Work out the finished part from the listing and answer in its coordinate system (mm). A direction names the side the tool comes from. Give positions to 0.01 mm unless a question says otherwise; leave off trailing zeros. Loops run counter-clockwise (first coordinate to the right, second up) from the corner with the lowest first, then second, coordinate; pieces in that order, holes last. Notation, with made-up numbers: M -24,-25 L 17,-25 A19 cw 17,-4 Z; hole C -21,82 d8. An arc over 180 degrees is marked long. Answer in a Markdown table with one row per item. Add a question column.
from build123d import *

# Parameters (mm, degrees)
BOSS_EXTRUDE1_DEPTH      = 28.5
SKETCH2_W                = 12
SKETCH2_H                = 11
SKETCH2_R                = 1.7
BOSS_EXTRUDE2_DEPTH      = 3
SKETCH3_W                = 19
SKETCH3_H                = 6
BOSS_EXTRUDE3_DEPTH      = 4
M3_CLEARANCE_HOLE1_D     = 3.2
M3_CLEARANCE_HOLE1_DEPTH = 4
FILLET1_R                = 3
M3_CLEARANCE_HOLE2_D     = 3.6
FILLET2_R                = 2


with BuildPart() as part:
    # Sketch1 → Boss-Extrude1 (new body)
    with BuildSketch(Plane.XY):
        with BuildLine():
            Line((-3.5, 44), (-3.5, 39.846580782))
            ThreePointArc((-3.5, 39.846580782), (0, 40), (3.5, 39.846580782))
            Line((3.5, 39.846580782), (3.5, 44))
            Line((3.5, 44), (-3.5, 44))
        make_face()
    extrude(amount=BOSS_EXTRUDE1_DEPTH)

    # Sketch2 → Boss-Extrude2 (add)
    with BuildSketch(Plane(origin=(0, 0, 0), x_dir=(-1, 0, 0), z_dir=(0, 0, -1))):
        with Locations((0, 38.5)):
            Rectangle(SKETCH2_W, SKETCH2_H)
        with Locations((-3.137606739, 35.863009131)):
            Circle(SKETCH2_R, mode=Mode.SUBTRACT)
        with Locations((3.137606739, 35.863009131)):
            Circle(SKETCH2_R, mode=Mode.SUBTRACT)
    extrude(amount=BOSS_EXTRUDE2_DEPTH)

    # Sketch3 → Boss-Extrude3 (add)
    with BuildSketch(Plane.XY.offset(28.5)):
        with Locations((0, 41)):
            Rectangle(SKETCH3_W, SKETCH3_H)
    extrude(amount=-BOSS_EXTRUDE3_DEPTH)

    # M3 Clearance Hole1
    with Locations(Plane.XY.offset(28.5)):
        with Locations((-6.25, 41), (6.25, 41)):
            Hole(M3_CLEARANCE_HOLE1_D / 2, depth=M3_CLEARANCE_HOLE1_DEPTH)

    # Fillet1
    fillet1_edges = [part.edges().sort_by_distance(p)[0] for p in [
        (9.5, 38, 26.5),
        (9.5, 44, 26.5),
        (-9.5, 38, 26.5),
        (-9.5, 44, 26.5),
    ]]
    fillet(fillet1_edges, radius=FILLET1_R - 0.0001)  # a hair under: the kernel refuses the full size

    # M3 Clearance Hole2 (through all)
    with Locations(Plane(origin=(0, 44, 0), x_dir=(1, 0, 0), z_dir=(0, 1, 0))):
        with Locations((0, -20)):
            Hole(M3_CLEARANCE_HOLE2_D / 2)

    # Fillet2
    fillet2_edges = [part.edges().sort_by_distance(p)[0] for p in [
        (6, 44, -1.5),
        (-6, 44, -1.5),
    ]]
    fillet(fillet2_edges, radius=FILLET2_R)


solid = part.part
(1) Section B-B, the plane y = 40.5 is taken. Determine the outline of the cut face in (x, z), and give its area (3 significant figures).
(2) Section D-D, the plane x = 3 is taken. Determine the outline of the cut face in (y, z), and give its area (3 significant figures).
(3) Consider line 1 along Z through (x, y) = (0, 41.85); line 2 along Y through (x, z) = (-6.25, 25.35); line 3 along X through (y, z) = (42.35, 20). Determine where each line is inside the solid, lowest interval first. Write a range as from..to.
(4) Section C-C, the plane y = 34.5 is taken. Determine the outline of the cut face in (x, z).
(5) Each of these flat-tipped pins is pushed along its axis until it touches: P1, Ø6, axis at x = 0, z = 20, coming from the -Y side; P2, Ø3, axis at x = -3.14, y = 35.86, coming from the -Z side; P3, Ø2, axis at x = 2, z = 26, coming from the -Y side; P4, Ø1.5, axis at y = 37, z = -1.5, coming from the +X side. Where does it stop, or does it pass through?
(6) Which of the six approach directions +Z, -Z, +X, -X, +Y, -Y give full straight-line access (tool end or side, diameter ignored) to faces 1 (the face through (0, 38, 27)), 2 (the face through (-3.5, 42, 12)), 3 (the face through (0, 40, 12)), 4 (the face through (5.51, 39.58, 26.47)), 5 (the face through (5.4, 43.43, -1.52))?
(7) The mould has two halves that part along Z. Classify faces 6 (the face through (3.5, 42, 12)), 7 (the face through (8.6, 43.14, 26.47)), 8 (the face through (0, 39, -3)), 9 (the face through (-0.1, 39.7, 24.5)): pulls with the +Z half, pulls with the -Z half, needs draft (parallel to the pull), parting line crosses it, or undercut.
(8) Section A-A, the plane z = 20 is taken. Determine the outline of the cut face in (x, y).
Numbers:
| question | item | result |
|---|---|---|
| 1 | outline | M -9.46,24.5 L -7.77,24.5 L -7.77,28.5 L -9.46,28.5 Z; M -6,-3 L 6,-3 L 6,0 L 3.5,0 L 3.5,24.5 L 4.73,24.5 L 4.73,28.5 L -4.73,28.5 L -4.73,24.5 L -3.5,24.5 L -3.5,0 L -6,0 Z; M 7.77,24.5 L 9.46,24.5 L 9.46,28.5 L 7.77,28.5 Z; hole C 0,20 d3.6 |
| 1 | area | 249 mm² |
| 2 | outline | M 33,-3 L 34.17,-3 L 34.17,0 L 33,0 Z; M 37.56,-3 L 44,-3 L 44,28.5 L 38,28.5 L 38,24.5 L 39.89,24.5 L 39.89,0 L 37.56,0 Z |
| 2 | area | 148 mm² |
| 3 | line 1 | z = -3..18.2, 21.8..28.5 |
| 3 | line 2 | y = 38..39.4, 42.6..44 |
| 3 | line 3 | x = -3.5..-1.8, 1.8..3.5 |
| 4 | outline | M -6,-3 L -4.15,-3 L -4.15,0 L -6,0 Z; M -2.12,-3 L 2.12,-3 L 2.12,0 L -2.12,0 Z; M 4.15,-3 L 6,-3 L 6,0 L 4.15,0 Z |
| 5 | P1 | stops at y = 39.89 |
| 5 | P2 | passes through |
| 5 | P3 | stops at y = 38 |
| 5 | P4 | stops at x = 6 |
| 6 | face 1 | +Z, +X, -X, -Y |
| 6 | face 2 | -X, +Y, -Y |
| 6 | face 3 | -Y |
| 6 | face 4 | +Z |
| 6 | face 5 | -Z, +X, +Y |
| 7 | face 6 | undercut |
| 7 | face 7 | needs draft |
| 7 | face 8 | pulls with the -Z half |
| 7 | face 9 | undercut |
| 8 | outline | M -3.5,39.85 A40 cw -1.8,39.96 L -1.8,44 L -3.5,44 Z; M 1.8,39.96 A40 cw 3.5,39.85 L 3.5,44 L 1.8,44 Z |
